Build history of the part. All positions in model axes, mm. A direction names the side the tool comes from. Coordinates: 2 decimals unless noted, no trailing zeros. Write each loop counter-clockwise with the first axis right and the second up, starting at its lowest first coordinate (ties: lowest second). Pieces come first, ordered by that corner, then holes.
```python
from build123d import *

# Parameters (mm, degrees)
BOSS_EXTRUDE1_DEPTH = 70
CUT_EXTRUDE1_DEPTH  = 65
SKETCH5_R           = 8.5
CUT_EXTRUDE2_DEPTH  = 10
SKETCH6_R           = 8.5
CUT_EXTRUDE3_DEPTH  = 10
CHAMFER2_SIZE       = 1
SKETCH7_W           = 11
SKETCH7_H           = 11
CUT_EXTRUDE4_DEPTH  = 10
SKETCH8_W           = 11
SKETCH8_H           = 11
CUT_EXTRUDE5_DEPTH  = 10
SKETCH9_W           = 15
SKETCH9_H           = 10
BOSS_EXTRUDE2_DEPTH = 6
FILLET1_R           = 8
FILLET2_R           = 4
SKETCH11_R          = 2.484902638
CUT_EXTRUDE7_DEPTH  = 10


with BuildPart() as part:
    # Sketch1 → Boss-Extrude1 (new body)
    with BuildSketch(Plane(origin=(0, 0, 0), x_dir=(1, 0, 0), z_dir=(0, 1, 0))):
        Polygon((-55.37403033, -102.482648945), (3.252686078, -116.449526131), (57.060212297, -100.408827863), (76.3, -57.735026919), (-76.3, -57.735026919), align=None)
    extrude(amount=BOSS_EXTRUDE1_DEPTH)

    # Sketch4 → Cut-Extrude1 (cut)
    with BuildSketch(Plane(origin=(0, 70, 0), x_dir=(1, 0, 0), z_dir=(0, 1, 0))):
        Polygon((-51.867290581, -98.178143042), (3.108154981, -111.275163368), (53.44146669, -96.270172009), (71.3, -57.735026919), (-71.3, -57.735026919), align=None)
    extrude(amount=-CUT_EXTRUDE1_DEPTH, mode=Mode.SUBTRACT)

    # Sketch5 → Cut-Extrude2 (cut)
    with BuildSketch(Plane(origin=(-26.077584107, 0, 109.462058529), x_dir=(0.9727757912880333, 0, 0.23174826835154788), z_dir=(-0.23174826835154788, 0, 0.9727757912880333))):
        with Locations((10.114141871, 42.998978407)):
            Circle(SKETCH5_R)
        with Locations((9.883660258, 17)):
            Circle(SKETCH5_R)
    extrude(amount=-CUT_EXTRUDE2_DEPTH, mode=Mode.SUBTRACT)

    # Sketch6 → Cut-Extrude3 (cut)
    with BuildSketch(Plane(origin=(32.147178959, 0, 107.83571549), x_dir=(0.9583226816177197, 0, -0.28568800796852273), z_dir=(0.2856880079685227, 0, 0.9583226816177196))):
        with Locations((-10.151110305, 17)):
            Circle(SKETCH6_R)
        with Locations((-10.151110305, 43)):
            Circle(SKETCH6_R)
    extrude(amount=-CUT_EXTRUDE3_DEPTH, mode=Mode.SUBTRACT)

    # Chamfer2
    chamfer2_edges = [part.edges().sort_by_distance(p)[0] for p in [
        (-24.507385971, 42.998978407, 109.836133113),
        (-24.731592905, 17, 109.782719398),
        (14.273396917, 17, 113.164114039),
        (14.273396917, 43, 113.164114039),
    ]]
    chamfer(chamfer2_edges, length=CHAMFER2_SIZE)

    # Sketch7 → Cut-Extrude4 (cut)
    with BuildSketch(Plane(origin=(-26.077584107, 0, 109.462058529), x_dir=(0.9727757912880333, 0, 0.23174826835154788), z_dir=(-0.23174826835154788, 0, 0.9727757912880333))):
        with Locations((-14.616339742, 28)):
            Rectangle(SKETCH7_W, SKETCH7_H)
    extrude(amount=-CUT_EXTRUDE4_DEPTH, mode=Mode.SUBTRACT)

    # Sketch8 → Cut-Extrude5 (cut)
    with BuildSketch(Plane(origin=(32.147178959, 0, 107.83571549), x_dir=(0.9583226816177197, 0, -0.28568800796852273), z_dir=(0.2856880079685227, 0, 0.9583226816177196))):
        with Locations((10.496497648, 28)):
            Rectangle(SKETCH8_W, SKETCH8_H)
    extrude(amount=-CUT_EXTRUDE5_DEPTH, mode=Mode.SUBTRACT)

    # Sketch9 → Boss-Extrude2 (add)
    with BuildSketch(Plane(origin=(0, 0, 57.735026919), x_dir=(-1, 0, 0), z_dir=(0, 0, -1))):
        with Locations((0, 10)):
            Rectangle(SKETCH9_W, SKETCH9_H)
    extrude(amount=-BOSS_EXTRUDE2_DEPTH)

    # Fillet1
    # the kernel refuses this fillet: 8 mm, written as the material it takes off along each edge
    with BuildSketch(Plane(origin=(-7.5, 15, 37.735026919), x_dir=(0, -1, 0), z_dir=(0, 0, 1))) as fillet1_piece_1:
        with BuildLine():
            CenterArc((FILLET1_R, FILLET1_R), FILLET1_R, 180, 90)
            Line((0, FILLET1_R), (0, 0))
            Line((0, 0), (FILLET1_R, 0))
        make_face()
    extrude(amount=46, mode=Mode.SUBTRACT)
    with BuildSketch(Plane(origin=(7.5, 15, 37.735026919), x_dir=(0, -1, 0), z_dir=(0, 0, 1))) as fillet1_piece_2:
        with BuildLine():
            CenterArc((FILLET1_R, -FILLET1_R), FILLET1_R, 90, 90)
            Line((0, -FILLET1_R), (0, 0))
            Line((0, 0), (FILLET1_R, 0))
        make_face()
    extrude(amount=46, mode=Mode.SUBTRACT)

    # Fillet2
    # the kernel refuses this fillet: 4 mm, written as the material it adds along each edge
    with BuildSketch(Plane(origin=(-7.5, 5, 57.735026919), x_dir=(-1, 0, 0), z_dir=(0, 0, 1))) as fillet2_piece_1:
        with BuildLine():
            CenterArc((3.832159566, -4), FILLET2_R, 90, 80.405931773)
            Line((-0.111893623, -3.333333333), (-0.506298941, -3.266666667))
            ThreePointArc((-0.506298941, -3.266666667), (-0.4, -2), (-0.4, 0))
            Line((-0.4, 0), (0, 0.4))
            Line((0, 0.4), (3.832159566, 0.4))
            Line((3.832159566, 0.4), (3.832159566, 0))
        make_face()
    extrude(amount=6)
    with BuildSketch(Plane(origin=(7.5, 5, 57.735026919), x_dir=(1, 0, 0), z_dir=(0, 0, 1))) as fillet2_piece_2:
        with BuildLine():
            CenterArc((3.832159566, 4), FILLET2_R, 189.594068227, 80.405931773)
            Line((-0.111893623, 3.333333333), (-0.506298941, 3.266666667))
            ThreePointArc((-0.506298941, 3.266666667), (-0.4, 2), (-0.4, 0))
            Line((-0.4, 0), (0, -0.4))
            Line((0, -0.4), (3.832159566, -0.4))
            Line((3.832159566, -0.4), (3.832159566, 0))
        make_face()
    extrude(amount=6)

    # Sketch11 → Cut-Extrude7 (cut)
    with BuildSketch(Plane(origin=(0, 0, 57.735026919), x_dir=(-1, 0, 0), z_dir=(0, 0, -1))):
        with Locations((0, 9)):
            Circle(SKETCH11_R)
    extrude(amount=-CUT_EXTRUDE7_DEPTH, mode=Mode.SUBTRACT)


solid = part.part
```
1. Saw through at C-C on x = 18.5. State how many separate pieces and enclosed holes the cut face has, plus the area to 3 significant figures.
Computed values:
separate pieces: 3
enclosed holes: 0
area: 445 mm2
2. Flat gauge pins, fed straight in: pin 1 (5 mm diameter, centred on x = 37, y = 45.5, fed in from -Z); pin 2 (4 mm diameter, centred on x = -9.5, z = 87, fed in from +Y); pin 3 (10 mm diameter, centred on x = -35, y = 17.5, fed in from +Z). Where does each tip first touch, or does it go through?
Computed values:
pin 1: stops at z = 100.43
pin 2: stops at y = 5
pin 3: stops at z = 108.53
3. 3-axis set-ups, long thin cutter, end or side, ignore diameter. For faces 4 (the face through (-61.72, 37.96, 77.67)), 5 (the face through (-45.075, 27.923, 102.402)), 6 (the face through (36.231, 27.923, 104.046)): which of +Z, -Z, +X, -X, +Y, -Y reach the whole face in a straight line?
Computed values:
face 4: -Z, +Y
face 5: +Z
face 6: -Z
4. Mould opens along Z. For faces 1 (the face through (41, 33.5, 102)), 2 (the face through (-1, 5, 78)), 3 (the face through (-16.626, 51.427, 108.658)) say: +Z half, -Z half, draft (parallel to the pull), parting line (faces both ways), or undercut.
Computed values:
face 1: draft
face 2: undercut
face 3: parting line
5. Probe line 1 along Y through (x, z) = (0, 61.9); line 2 along Y through (x, z) = (-36, 98.5); line 3 along X through (y, z) = (30, 89.5). List the from-to ranges inside material, lowest first.
Computed values:
line 1: y = 0 to 6.52, 11.48 to 14.98
line 2: y = 0 to 5
line 3: x = -61.45 to -56.04, 56.58 to 61.98
6. Saw through at A-A on y = 32. List the corners of the cut face in (x, z).
Computed values:
outline: (-76.3, 57.74) - (-71.3, 57.74) - (-51.87, 98.18) - (-44.49, 99.94) - (-45.65, 104.8) - (-55.37, 102.48) - close; (-34.95, 107.35) - (-33.79, 102.49) - (3.11, 111.28) - (35.51, 101.62) - (36.94, 106.41) - (3.25, 116.45) - close; (46.05, 98.47) - (53.44, 96.27) - (71.3, 57.74) - (76.3, 57.74) - (57.06, 100.41) - (47.48, 103.27) - close
7. Saw through at B-B on z = 75. List the corners of the cut face in (x, y), plus the area to 3 significant figures.
Computed values:
outline: (-68.23, 0) - (68.52, 0) - (68.52, 70) - (63.3, 70) - (63.3, 5) - (-63, 5) - (-63, 70) - (-68.23, 70) - close
area: 1,360 mm2
